Study the drawing (mm; zero at the part's minimum x, y, z) and answer. Coordinates: 2 decimals unless noted, no trailing zeros. Order: outer loops, then holes, each group sorted by start corner. A loop starts at its lowest first (then second) coordinate and runs counter-clockwise, first axis right, second up. Notation, with made-up numbers: (42.5, 0) -> (80.5, 0) arc R35 ccw to (80.5, 35) -> close; hole circle Ø7 at (18.5, 50.5). An arc over 180 degrees is marked (long way). Write each question's results on one line, items separated by ' | '. Start each with the question number.
(1) The part is cut by section A-A, the plane y = 141. Give the vertices of the cut face in (x, z).
(2) The part is cut by section C-C, the plane y = 36. Give the vertices of the cut face in (x, z), then the cut area to 3 significant figures.
(3) The part is cut by section B-B, the plane z = 2. Give the vertices of the cut face in (x, y), then the cut area to 3 significant figures.
(4) The part is cut by section D-D, the plane x = 42. Give the vertices of the cut face in (y, z), then the cut area to 3 significant figures.
(5) Straight lines are drawn through the part: L1, parallel to X at y = 119, z = 4.2; L2, parallel to X at y = 108, z = 3; L3, parallel to Y at x = 165, z = 3.05. For each, find the intervals that lie inside material, in ascending order.
(6) Given pin 1 (3 mm diameter, centred on x = 88.5, z = 1, fed in from -Y); pin 2 (3 mm diameter, centred on y = 3.5, z = 4.5, fed in from +X); pin 3 (1.8 mm diameter, centred on y = 11, z = 4, fed in from -X), each flat-ended and moving along its own axis, determine where each tip first touches the part or whether it passes through.
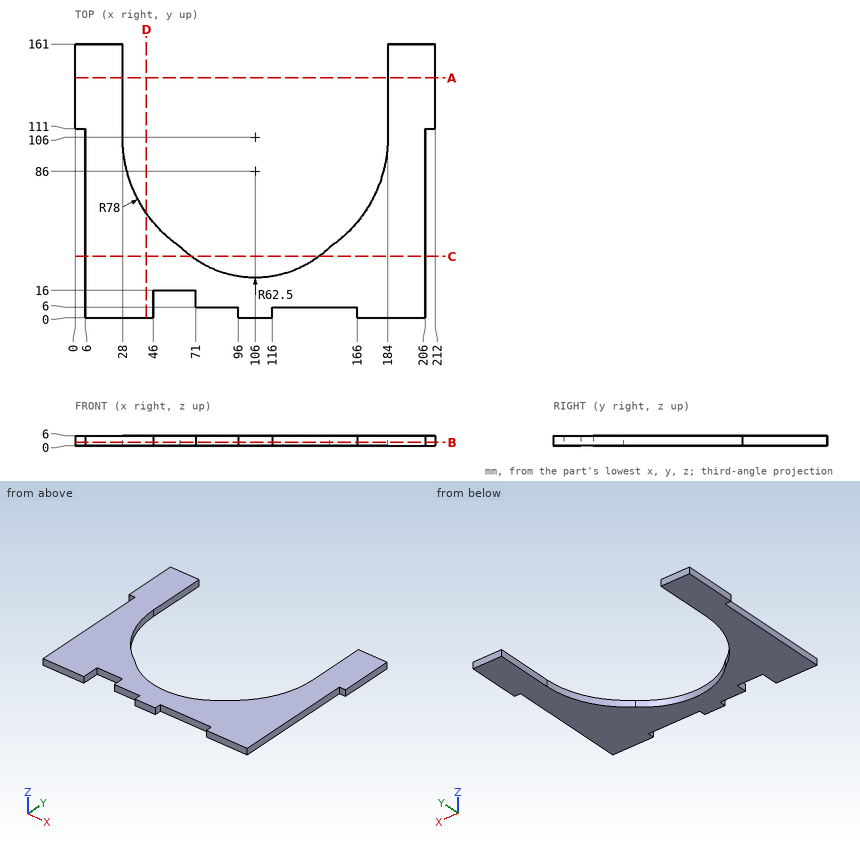
Established:
1) outline: (0, 0) -> (28, 0) -> (28, 6) -> (0, 6) -> close; (184, 0) -> (212, 0) -> (212, 6) -> (184, 6) -> close
2) outline: (6, 0) -> (68.5, 0) -> (68.5, 6) -> (6, 6) -> close; (143.5, 0) -> (206, 0) -> (206, 6) -> (143.5, 6) -> close | area: 750 mm^2
3) outline: (0, 111) -> (6, 111) -> (6, 0) -> (46, 0) -> (46, 16) -> (71, 16) -> (71, 6) -> (96, 6) -> (96, 0) -> (116, 0) -> (116, 6) -> (166, 6) -> (166, 0) -> (206, 0) -> (206, 111) -> (212, 111) -> (212, 161) -> (184, 161) -> (184, 106) arc R78 cw to (149.94, 41.56) arc R62.5 cw to (62.06, 41.56) arc R78 cw to (28, 106) -> (28, 161) -> (0, 161) -> close | area: 13,500 mm^2
4) outline: (0, 0) -> (61.41, 0) -> (61.41, 6) -> (0, 6) -> close | area: 368 mm^2
5) L1: x = 0 to 28, 184 to 212 | L2: x = 6 to 28, 184 to 206 | L3: y = 6 to 54.98
6) pin 1: stops at y = 6 | pin 2: stops at x = 206 | pin 3: stops at x = 6
